from build123d import *

# Parameters (mm, degrees)
SKETCH1_W           = 92.1
SKETCH1_H           = 14.3
BOSS_EXTRUDE1_DEPTH = 3.175
SKETCH2_W           = 10
SKETCH2_H           = 3.175
BOSS_EXTRUDE2_DEPTH = 3.175
SKETCH3_W           = 8
SKETCH3_H           = 3.175
BOSS_EXTRUDE3_DEPTH = 3.175


with BuildPart() as part:
    # Sketch1 → Boss-Extrude1 (new body)
    with BuildSketch(Plane(origin=(0, 0, 0), x_dir=(1, 0, 0), z_dir=(0, 1, 0))):
        Rectangle(SKETCH1_W, SKETCH1_H)
    extrude(amount=BOSS_EXTRUDE1_DEPTH)

    # Sketch2 → Boss-Extrude2 (add)
    with BuildSketch(Plane(origin=(0, 0, -7.15), x_dir=(-1, 0, 0), z_dir=(0, 0, -1))):
        with Locations((-33.05, 1.5875)):
            Rectangle(SKETCH2_W, SKETCH2_H)
        with Locations((33.05, 1.5875)):
            Rectangle(SKETCH2_W, SKETCH2_H)
    extrude(amount=BOSS_EXTRUDE2_DEPTH)

    # Sketch3 → Boss-Extrude3 (add)
    with BuildSketch(Plane.ZY.offset(46.05)):
        with Locations((0, 1.5875)):
            Rectangle(SKETCH3_W, SKETCH3_H)
    boss_extrude3 = extrude(amount=BOSS_EXTRUDE3_DEPTH)

    # Mirror1: Boss-Extrude3 across plane
    add(boss_extrude3.mirror(Plane(origin=(0, 0, 0), x_dir=(0, 0, 1), z_dir=(1, 0, 0))))


solid = part.part
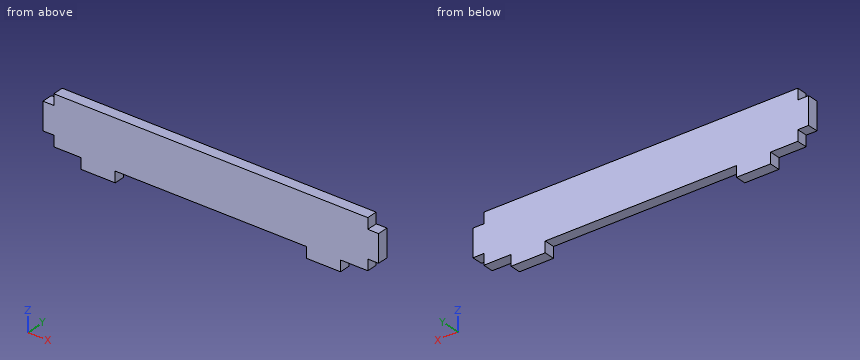
For this review, take the finished solid that the model builds, in its own axes (mm). Round coordinates to 2 decimals unless told otherwise and drop trailing zeros. Write each loop counter-clockwise with the first axis right and the second up, starting at its lowest first coordinate (ties: lowest second). Pieces come first, ordered by that corner, then holes. Notation, with made-up numbers: (60.5, 11.5) - (105.5, 11.5) arc R16 cw to (105.5, 39.5) - close; hole circle Ø4 at (-12, 55). An arc over 180 degrees is marked (long way). Write item = value, one per line. Start each with the question number.
1. Wall thickness on L1, parallel to X at y = 0.7, z = -8.5; L2, parallel to Z at x = -44.5, y = 0.75; L3, parallel to X at y = 0.65, z = 5.5: over which ranges is each line inside the solid? List them lowest first.
2. Consider section A-A on z = -8. State the section outline as (x, y) points (3 decimals), plus the area to 3 significant figures.
3. Consider section B-B on y = 1. State the section outline as (x, z) points (3 decimals).
4. For pin 1 Ø1.6 at (y, z) = (1.5, 5.5) entering from -X; pin 2 Ø1.5 at (x, y) = (15, 0.5) entering from -Z; pin 3 Ø1 at (x, y) = (-48, 1) entering from -Z, all flat-tipped, find the tip position at first contact; note any pin that passes through.
5. Consider section C-C on z = 5. State the section outline as (x, y) points (3 decimals), plus the area to 3 significant figures.
6. Consider section D-D on x = -7. State the section outline as (y, z) points (3 decimals), plus the area to 3 significant figures.
Evaluation:
q1.L1 = -38.05 to -28.05, 28.05 to 38.05
q1.L2 = -7.15 to 7.15
q1.L3 = -46.05 to 46.05
q2.outline = (-38.05, 0) - (-28.05, 0) - (-28.05, 3.175) - (-38.05, 3.175) - close; (28.05, 0) - (38.05, 0) - (38.05, 3.175) - (28.05, 3.175) - close
q2.area = 63.5 mm2
q3.outline = (-49.225, -4) - (-46.05, -4) - (-46.05, -7.15) - (-38.05, -7.15) - (-38.05, -10.325) - (-28.05, -10.325) - (-28.05, -7.15) - (28.05, -7.15) - (28.05, -10.325) - (38.05, -10.325) - (38.05, -7.15) - (46.05, -7.15) - (46.05, -4) - (49.225, -4) - (49.225, 4) - (46.05, 4) - (46.05, 7.15) - (-46.05, 7.15) - (-46.05, 4) - (-49.225, 4) - close
q4.pin_1 = -46.05
q4.pin_2 = -7.15
q4.pin_3 = -4
q5.outline = (-46.05, 0) - (46.05, 0) - (46.05, 3.175) - (-46.05, 3.175) - close
q5.area = 292 mm2
q6.outline = (0, -7.15) - (3.175, -7.15) - (3.175, 7.15) - (0, 7.15) - close
q6.area = 45.4 mm2
